The model under review builds one solid part; all positions refer to its coordinate system, in mm. Face numbers are marked on the shaded views. A direction names the side the tool comes from. Coordinates: 2 decimals unless noted, no trailing zeros. Order: outer loops, then holes, each group sorted by start corner. A loop starts at its lowest first (then second) coordinate and runs counter-clockwise, first axis right, second up. Notation, with made-up numbers: (44.25, 76) - (85.25, 76) arc R25 ccw to (85.25, 96) - close; hole circle Ø1 at (-22, -8). An arc over 180 degrees is marked (long way). Answer in a Markdown table with one row per item.
```python
from build123d import *

# Parameters (mm, degrees)
F0_W           = 32.4746801579
F0_H           = 12.0628447294
F1_DEPTH       = 4
F2_D           = 2.5
F2_DEPTH       = 13.5
F2_CBORE_D     = 6.5
F2_CBORE_DEPTH = 3
F2_TIP         = 0.7510757738
F3_W           = 32.4746801579
F3_H           = 4
F3_H_2         = 32
F3_R           = 11
F4_DEPTH       = 4


with BuildPart() as f1:
    # F0 (on Top) → F1 (new body)
    with BuildSketch(Plane.XY):
        Rectangle(F0_W, F0_H)
    extrude(amount=F1_DEPTH)

    # F2
    with Locations(Plane(origin=(0, 0, 0), x_dir=(1, 0, 0), z_dir=(0, 0, -1))):
        with Locations((10.0235303257, 0), (-9.9764696743, 0)):
            CounterBoreHole(F2_D / 2, F2_CBORE_D / 2, F2_CBORE_DEPTH, depth=F2_DEPTH)
            with Locations((0, 0, -(F2_DEPTH + F2_TIP / 2))):  # 118° drill point
                Cone(0, F2_D / 2, F2_TIP, mode=Mode.SUBTRACT)

    # F3 (on face) → F4 (join)
    with BuildSketch(Plane(origin=(0, 6.0314223647, 0), x_dir=(-1, 0, 0), z_dir=(0, 1, 0))):
        with Locations((0, 2)):
            Rectangle(F3_W, F3_H)
        with Locations((0, -16)):
            Rectangle(F3_W, F3_H_2)
        with Locations((0, -16)):
            Circle(F3_R, mode=Mode.SUBTRACT)
    extrude(amount=F4_DEPTH)


solid = f1.part
```
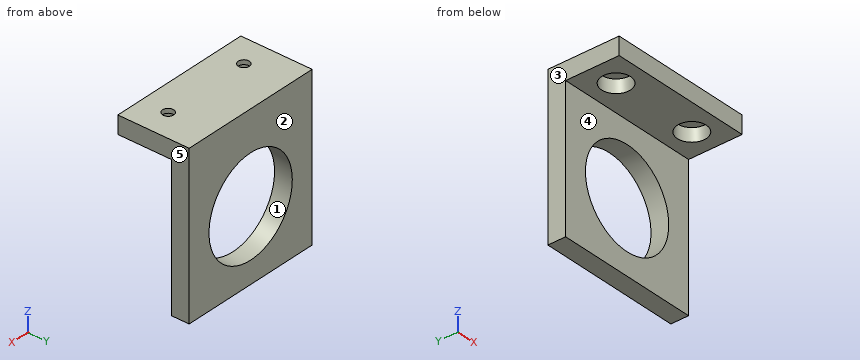
Item 1: We need section B-B, the plane y = 0. Write out the cut boundary in (x, z).
Check values:
| item | result |
|---|---|
| outline | (-16.24, 0) - (-13.23, 0) - (-13.23, 3) - (-11.23, 3) - (-11.23, 4) - (-16.24, 4) - close; (-8.73, 3) - (-6.73, 3) - (-6.73, 0) - (6.77, 0) - (6.77, 3) - (8.77, 3) - (8.77, 4) - (-8.73, 4) - close; (11.27, 3) - (13.27, 3) - (13.27, 0) - (16.24, 0) - (16.24, 4) - (11.27, 4) - close |
Item 2: Clearance check with flat-ended pins moving along their axes: pin 1 Ø2 at (x, y) = (8.5, 0.5) entering from -Z; pin 2 Ø1 at (x, z) = (-11, -22.5) entering from -Y; pin 3 Ø7.5 at (x, y) = (-9.98, 0) entering from +Z; pin 4 Ø3 at (x, y) = (-12.5, 4.5) entering from -Z. State where each tip first meets the part, or that it passes through.
Check values:
| item | result |
|---|---|
| pin 1 | z = 3 |
| pin 2 | y = 6.03 |
| pin 3 | z = 4 |
| pin 4 | z = 0 |
Item 3: Tool access review of the marked faces 4 and 5: name each direction out of +Z, -Z, +X, -X, +Y, -Y from which nothing blocks a thin tool from reaching the whole face with its end or side.
Check values:
| item | result |
|---|---|
| face 4 | -Z, +X, -X, -Y |
| face 5 | +Z, -Z, +X, +Y, -Y |
Item 4: Mouldability with a two-part tool opening along X and no side actions: class the marked faces 1, 2 and 3 as +X half, -X half, draft (parallel to the pull), parting line (faces both ways), or undercut.
Check values:
| item | result |
|---|---|
| face 1 | undercut |
| face 2 | draft |
| face 3 | -X half |
Item 5: We need section C-C, the plane z = -16. Write out the cut boundary in (x, y), then the cut area to 3 significant figures.
Check values:
| item | result |
|---|---|
| outline | (-16.24, 6.03) - (-11, 6.03) - (-11, 10.03) - (-16.24, 10.03) - close; (11, 6.03) - (16.24, 6.03) - (16.24, 10.03) - (11, 10.03) - close |
| area | 41.9 mm^2 |
Item 6: We need section D-D, the plane y = 7.75. Write out the cut boundary in (x, z), then the cut area to 3 significant figures.
Check values:
| item | result |
|---|---|
| outline | (-16.24, -32) - (16.24, -32) - (16.24, 4) - (-16.24, 4) - close; hole circle Ø22 at (0, -16) |
| area | 789 mm^2 |
Item 7: We need section A-A, the plane x = 0. Write out the cut boundary in (y, z).
Check values:
| item | result |
|---|---|
| outline | (-6.03, 0) - (6.03, 0) - (6.03, -5) - (10.03, -5) - (10.03, 4) - (-6.03, 4) - close; (6.03, -32) - (10.03, -32) - (10.03, -27) - (6.03, -27) - close |
Item 8: To check wall thickness, follow line 1 (Z direction, x = 0, y = 8); line 2 (Z direction, x = 13, y = 5); line 3 (Y direction, x = 10.5, z = -26.5). State the ranges of each line that lie inside material, in increasing order. Write a range as from..to.
Check values:
| item | result |
|---|---|
| line 1 | -32..-27, -5..4 |
| line 2 | 0..4 |
| line 3 | 6.03..10.03 |
